from build123d import *

# Parameters (mm, degrees)
BOSS_EXTRUDE1_DEPTH            = 5
FILLET1_R                      = 5
M5X0_8_TAPPED_HOLE1_AT_2_COUNT = 2
M5X0_8_TAPPED_HOLE1_AT_2_PITCH = 15
M5X0_8_TAPPED_HOLE1_AT_3_COUNT = 2
M5X0_8_TAPPED_HOLE1_AT_3_PITCH = 30
M5X0_8_TAPPED_HOLE1_AT_4_COUNT = 2
M5X0_8_TAPPED_HOLE1_AT_4_PITCH = 130
M5X0_8_TAPPED_HOLE1_AT_5_COUNT = 2
M5X0_8_TAPPED_HOLE1_AT_5_PITCH = 145
M5X0_8_TAPPED_HOLE1_AT_6_COUNT = 2
M5X0_8_TAPPED_HOLE1_AT_6_PITCH = 160


with BuildPart() as part:
    # Sketch1 → Boss-Extrude1 (new body, symmetric)
    with BuildSketch(Plane(origin=(0, 0, 0), x_dir=(1, 0, 0), z_dir=(0, 1, 0))):
        Polygon((-112.7, 139), (112.7, 139), (112.7, 84.857864376), (82.7, 54.857864376), (82.7, -54.857864376), (112.7, -84.857864376), (112.7, -139), (-112.7, -139), (-112.7, -84.857864376), (-82.7, -54.857864376), (-82.7, 54.857864376), (-112.7, 84.857864376), align=None)
        Polygon((11.942135624, 104.857864376), (57.3, 59.5), (11.942135624, 14.142135624), align=None, mode=Mode.SUBTRACT)
        Polygon((11.942135624, 119), (57.3, 119), (57.3, 73.642135624), align=None, mode=Mode.SUBTRACT)
        Polygon((82.7, 129), (102.7, 129), (102.7, 89), (82.7, 69), align=None, mode=Mode.SUBTRACT)
        Polygon((57.3, 45.357864376), (11.942135624, 0), (57.3, -45.357864376), align=None, mode=Mode.SUBTRACT)
        Polygon((102.7, -89), (82.7, -69), (82.7, -129), (102.7, -129), align=None, mode=Mode.SUBTRACT)
        Polygon((57.3, -59.5), (11.942135624, -14.142135624), (11.942135624, -104.857864376), align=None, mode=Mode.SUBTRACT)
        Polygon((57.3, -119), (57.3, -73.642135624), (11.942135624, -119), align=None, mode=Mode.SUBTRACT)
        Polygon((-11.942135624, -119), (-57.3, -119), (-57.3, -73.642135624), align=None, mode=Mode.SUBTRACT)
        Polygon((-11.942135624, -14.142135624), (-11.942135624, -104.857864376), (-57.3, -59.5), align=None, mode=Mode.SUBTRACT)
        Polygon((-57.3, -45.357864376), (-11.942135624, 0), (-57.3, 45.357864376), align=None, mode=Mode.SUBTRACT)
        Polygon((-102.7, -129), (-102.7, -89), (-82.7, -69), (-82.7, -129), align=None, mode=Mode.SUBTRACT)
        Polygon((-11.942135624, 14.142135624), (-11.942135624, 104.857864376), (-57.3, 59.5), align=None, mode=Mode.SUBTRACT)
        Polygon((-82.7, 69), (-82.7, 129), (-102.7, 129), (-102.7, 89), align=None, mode=Mode.SUBTRACT)
        Polygon((-57.3, 73.642135624), (-11.942135624, 119), (-57.3, 119), align=None, mode=Mode.SUBTRACT)
    extrude(amount=BOSS_EXTRUDE1_DEPTH, both=True)

    # Fillet1
    fillet1_edges = [part.edges().sort_by_distance(p)[0] for p in [
        (-57.3, 0, -59.5),
        (-11.942135624, 0, -14.142135624),
        (-11.942135624, 0, -104.857864376),
        (-11.942135624, 0, 0),
        (-57.3, 0, -45.357864376),
        (-57.3, 0, 45.357864376),
        (-11.942135624, 0, -119),
        (-57.3, 0, -119),
        (-57.3, 0, -73.642135624),
        (-11.942135624, 0, 119),
        (-57.3, 0, 73.642135624),
        (-57.3, 0, 119),
        (-11.942135624, 0, 14.142135624),
        (-57.3, 0, 59.5),
        (-11.942135624, 0, 104.857864376),
        (-102.7, 0, 129),
        (-82.7, 0, 129),
        (-82.7, 0, 69),
        (-102.7, 0, 89),
        (-102.7, 0, -89),
        (-82.7, 0, -69),
        (-82.7, 0, -129),
        (-102.7, 0, -129),
        (112.7, 0, 84.857864376),
        (112.7, 0, 139),
        (-112.7, 0, 139),
        (-112.7, 0, 84.857864376),
        (-82.7, 0, 54.857864376),
        (-82.7, 0, -54.857864376),
        (-112.7, 0, -84.857864376),
        (-112.7, 0, -139),
        (112.7, 0, -139),
        (112.7, 0, -84.857864376),
        (82.7, 0, -54.857864376),
        (82.7, 0, 54.857864376),
        (11.942135624, 0, -104.857864376),
        (11.942135624, 0, -14.142135624),
        (57.3, 0, -59.5),
        (102.7, 0, 129),
        (102.7, 0, 89),
        (82.7, 0, 69),
        (82.7, 0, 129),
        (11.942135624, 0, -119),
        (57.3, 0, -73.642135624),
        (57.3, 0, -119),
        (11.942135624, 0, 104.857864376),
        (57.3, 0, 59.5),
        (11.942135624, 0, 14.142135624),
        (82.7, 0, -69),
        (102.7, 0, -89),
        (102.7, 0, -129),
        (82.7, 0, -129),
        (57.3, 0, 45.357864376),
        (57.3, 0, -45.357864376),
        (11.942135624, 0, 0),
        (11.942135624, 0, 119),
        (57.3, 0, 119),
        (57.3, 0, 73.642135624),
    ]]
    fillet(fillet1_edges, radius=FILLET1_R)

    # Sketch5 → M5x0.8 Tapped Hole1 (revolve, cut)
    with BuildSketch(Plane(origin=(80, 0, -139), x_dir=(0, 1, 0), z_dir=(1, 0, 0))):
        Polygon((0, 0), (0, 13.6618073), (2.1, 12.4), (2.1, 0), align=None)
    m5x0_8_tapped_hole1 = revolve(axis=Axis((80, 0, -145.35), (0, 0, 1)), mode=Mode.SUBTRACT)

    # M5x0.8 Tapped Hole1 at 2: M5x0.8 Tapped Hole1 ×2
    with Locations(*[(-i * M5X0_8_TAPPED_HOLE1_AT_2_PITCH, 0, 0) for i in range(1, M5X0_8_TAPPED_HOLE1_AT_2_COUNT)]):
        add(m5x0_8_tapped_hole1, mode=Mode.SUBTRACT)

    # M5x0.8 Tapped Hole1 at 3: M5x0.8 Tapped Hole1 ×2
    with Locations(*[(-i * M5X0_8_TAPPED_HOLE1_AT_3_PITCH, 0, 0) for i in range(1, M5X0_8_TAPPED_HOLE1_AT_3_COUNT)]):
        add(m5x0_8_tapped_hole1, mode=Mode.SUBTRACT)

    # M5x0.8 Tapped Hole1 at 4: M5x0.8 Tapped Hole1 ×2
    with Locations(*[(-i * M5X0_8_TAPPED_HOLE1_AT_4_PITCH, 0, 0) for i in range(1, M5X0_8_TAPPED_HOLE1_AT_4_COUNT)]):
        add(m5x0_8_tapped_hole1, mode=Mode.SUBTRACT)

    # M5x0.8 Tapped Hole1 at 5: M5x0.8 Tapped Hole1 ×2
    with Locations(*[(-i * M5X0_8_TAPPED_HOLE1_AT_5_PITCH, 0, 0) for i in range(1, M5X0_8_TAPPED_HOLE1_AT_5_COUNT)]):
        add(m5x0_8_tapped_hole1, mode=Mode.SUBTRACT)

    # M5x0.8 Tapped Hole1 at 6: M5x0.8 Tapped Hole1 ×2
    with Locations(*[(-i * M5X0_8_TAPPED_HOLE1_AT_6_PITCH, 0, 0) for i in range(1, M5X0_8_TAPPED_HOLE1_AT_6_COUNT)]):
        add(m5x0_8_tapped_hole1, mode=Mode.SUBTRACT)

    # Mirror1: M5x0.8 Tapped Hole1 across plane
    add(m5x0_8_tapped_hole1.mirror(Plane.XY), mode=Mode.SUBTRACT)

    # Mirror1 copy 1 sketch → Mirror1 copy 1 (revolve, cut)
    with BuildSketch(Plane(origin=(65, 0, 139), x_dir=(0, 1, 0), z_dir=(1, 0, 0))):
        Polygon((0, 0), (0, -13.6618073), (2.1, -12.4), (2.1, 0), align=None)
    revolve(axis=Axis((65, 0, 145.35), (0, 0, 1)), mode=Mode.SUBTRACT)

    # Mirror1 copy 2 sketch → Mirror1 copy 2 (revolve, cut)
    with BuildSketch(Plane(origin=(50, 0, 139), x_dir=(0, 1, 0), z_dir=(1, 0, 0))):
        Polygon((0, 0), (0, -13.6618073), (2.1, -12.4), (2.1, 0), align=None)
    revolve(axis=Axis((50, 0, 145.35), (0, 0, 1)), mode=Mode.SUBTRACT)

    # Mirror1 copy 3 sketch → Mirror1 copy 3 (revolve, cut)
    with BuildSketch(Plane(origin=(-50, 0, 139), x_dir=(0, 1, 0), z_dir=(1, 0, 0))):
        Polygon((0, 0), (0, -13.6618073), (2.1, -12.4), (2.1, 0), align=None)
    revolve(axis=Axis((-50, 0, 145.35), (0, 0, 1)), mode=Mode.SUBTRACT)

    # Mirror1 copy 4 sketch → Mirror1 copy 4 (revolve, cut)
    with BuildSketch(Plane(origin=(-65, 0, 139), x_dir=(0, 1, 0), z_dir=(1, 0, 0))):
        Polygon((0, 0), (0, -13.6618073), (2.1, -12.4), (2.1, 0), align=None)
    revolve(axis=Axis((-65, 0, 145.35), (0, 0, 1)), mode=Mode.SUBTRACT)

    # Mirror1 copy 5 sketch → Mirror1 copy 5 (revolve, cut)
    with BuildSketch(Plane(origin=(-80, 0, 139), x_dir=(0, 1, 0), z_dir=(1, 0, 0))):
        Polygon((0, 0), (0, -13.6618073), (2.1, -12.4), (2.1, 0), align=None)
    revolve(axis=Axis((-80, 0, 145.35), (0, 0, 1)), mode=Mode.SUBTRACT)


solid = part.part
Can you work these out from the model? Positions are in its coordinate system, mm. A direction names the side the tool comes from. Coordinates: 2 decimals unless noted, no trailing zeros. Write each loop counter-clockwise with the first axis right and the second up, starting at its lowest first coordinate (ties: lowest second). Pieces come first, ordered by that corner, then holes. Notation, with made-up numbers: M 76,62.25 L 106,62.25 A28 cw 106,101.25 Z; hole C 25.25,-12 d6. An arc over 180 degrees is marked long. Use one line per item in the form item = value.
Q1. I need wall thicknesses on line 1 along X through (y, z) = (0.5, -122); line 2 along Z through (x, y) = (54, -4); line 3 along X through (y, z) = (-3, 98.5). Which ranges of each line are inside material? Lowest first, please. Write a range as from..to.
Model answer:
line_1 = -112.7..-102.7, -82.7..82.7, 102.7..112.7
line_2 = -139..-118.7, -81.01..-62.78, -56.22..-37.99, 37.99..56.22, 62.78..81.01, 118.7..139
line_3 = -112.7..-102.7, -82.7..-57.3, -32.44..32.44, 57.3..82.7, 102.7..112.7
Q2. If we section it at C-C (z = 73): Write out the boundary of the cut face in (x, y).
Model answer:
outline = M -100.84,-5 L -43.8,-5 L -43.8,5 L -100.84,5 Z; M -11.94,-5 L 11.94,-5 L 11.94,5 L -11.94,5 Z; M 43.8,-5 L 100.84,-5 L 100.84,5 L 43.8,5 Z
Q3. If we section it at B-B (x = 28): Write out the boundary of the cut face in (y, z), then the cut area to 3 significant figures.
Model answer:
outline = M -5,-139 L 5,-139 L 5,-119 L -5,-119 Z; M -5,-102.94 L 5,-102.94 L 5,-88.8 L -5,-88.8 Z; M -5,-30.2 L 5,-30.2 L 5,-16.06 L -5,-16.06 Z; M -5,16.06 L 5,16.06 L 5,30.2 L -5,30.2 Z; M -5,88.8 L 5,88.8 L 5,102.94 L -5,102.94 Z; M -5,119 L 5,119 L 5,139 L -5,139 Z
area = 966 mm^2
Q4. If we section it at A-A (z = -7): Write out the boundary of the cut face in (x, y).
Model answer:
outline = M -82.7,-5 L -57.3,-5 L -57.3,5 L -82.7,5 Z; M -18.94,-5 L 18.94,-5 L 18.94,5 L -18.94,5 Z; M 57.3,-5 L 82.7,-5 L 82.7,5 L 57.3,5 Z
Q5. For P1, Ø4, axis at x = 65, y = 0, coming from the -Z side; P2, Ø4, axis at y = 4, z = -35, coming from the +X side; P3, Ø3.5, axis at x = -50, y = 0, coming from the +Z side, each with a flat end and sliding along its axis, tell me the tip position at first contact or that it passes through.
Model answer:
P1 = -126.54
P2 = 82.7
P3 = 126.39
Q6. We'd pull the mould along X, two halves only. Please class faces 1 (the cylindrical face through (19.363, 0.07, 115.837)), 2 (the flat face through (2, -5, -2)), 3 (the flat face through (-97.89, 0.07, 70.05)), 4 (the flat face through (57.3, 0, -100)): +X half, -X half, draft (parallel to the pull), parting line (faces both ways), or undercut.
Model answer:
face_1 = undercut
face_2 = draft
face_3 = -X half
face_4 = undercut
Q7. For faces 5 (the flat face through (-97.51, 0.07, -69.67)), 6 (the flat face through (-37.4, 0.1, -39.6)), 7 (the flat face through (-112.7, 0, 111)), which set-ups out of +Z, -Z, +X, -X, +Y, -Y let a thin tool reach every point of the face, with its end or its side?
Model answer:
face_5 = -X, +Y, -Y
face_6 = +Y, -Y
face_7 = +Z, -Z, -X, +Y, -Y
